Source: CAD feature listing. Evaluate the final solid. Frame: model axes, mm. Face numbers are marked on the shaded views. A direction names the side the tool comes from. Give positions to 0.01 mm unless a question says otherwise; leave off trailing zeros. Loops run counter-clockwise (first coordinate to the right, second up) from the corner with the lowest first, then second, coordinate; pieces in that order, holes last. Notation, with made-up numbers: M 59.5,42 L 94.5,42 A28 ccw 94.5,75 Z; hole C 82,59.25 d8. An arc over 180 degrees is marked long. Put each result on its own line as item: value.
from build123d import *

# Parameters (mm, degrees)
F1_DEPTH = 5
F3_DEPTH = 25


with BuildPart() as f1:
    # F0 (on Front) → F1 (new body)
    with BuildSketch(Plane.XZ):
        Polygon((48.04658, 78.242314), (-66.45342, 78.242314), (-66.45342, -34.757686), (-41.95342, -57.257686), (23.54658, -57.257686), (48.04658, -34.757686), align=None)
    extrude(amount=F1_DEPTH)

    # F2 (on face) → F3 (join)
    with BuildSketch(Plane.XZ.offset(5)):
        Polygon((23.54658, -57.257686), (48.04658, -34.757686), (48.04658, 78.242314), (-66.45342, 78.242314), (-66.45342, -34.757686), (-41.95342, -57.257686), align=None)
        Polygon((-61.45342, -32.560932), (-61.45342, 73.242314), (43.04658, 73.242314), (43.04658, -32.560932), (21.599003, -52.257686), (-40.005844, -52.257686), align=None, mode=Mode.SUBTRACT)
    extrude(amount=F3_DEPTH)


solid = f1.part
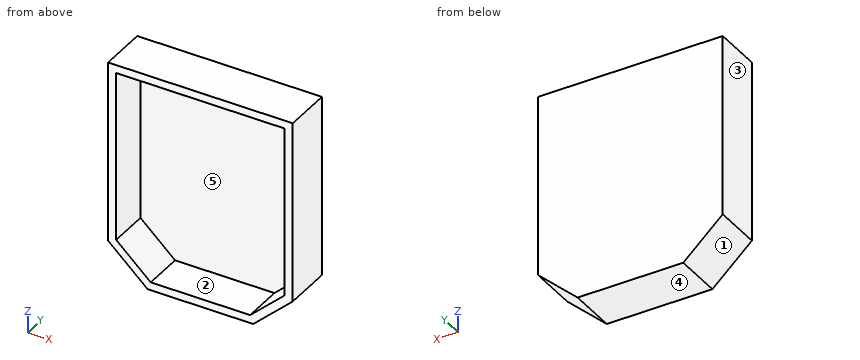
1. Section query A-A (y = -15.25). Output: boundary loops of the cut face in (x, z), plus the area to 3 significant figures.
Found:
outline: M -66.45,-34.76 L -41.95,-57.26 L 23.55,-57.26 L 48.05,-34.76 L 48.05,78.24 L -66.45,78.24 Z; hole M -61.45,-32.56 L -40.01,-52.26 L 21.6,-52.26 L 43.05,-32.56 L 43.05,73.24 L -61.45,73.24 Z
area: 2,270 mm^2
2. Section query B-B (x = -29). Output: boundary loops of the cut face in (y, z).
Found:
outline: M -30,-57.26 L 0,-57.26 L 0,78.24 L -30,78.24 L -30,73.24 L -5,73.24 L -5,-52.26 L -30,-52.26 Z
3. Contact query for a flat-ended pin moving along its axis: P1, Ø1, axis at x = 22.5, z = -10, coming from the -Y side. Output: stop coordinate, or through.
Found:
P1: y = -5
4. Material intervals for line 1 (Z direction, x = -39, y = -24.5); line 2 (X direction, y = -16, z = 23); line 3 (Y direction, x = -35, z = 60.5), sorted ascending. Write a range as from..to.
Found:
line 1: -57.26..-52.26, 73.24..78.24
line 2: -66.45..-61.45, 43.05..48.05
line 3: -5..0
5. Draft query along Z for the marked faces 3, 4 and 5. Return one class per face: pulls with the +Z half, pulls with the -Z half, needs draft (parallel to the pull), parting line crosses it, or undercut.
Found:
face 3: needs draft
face 4: pulls with the -Z half
face 5: undercut
6. Access query for the marked faces 1 and 2. Directions: +Z, -Z, +X, -X, +Y, -Y. A direction counts if a zero-diameter tool reaches every point of the face in a straight line with its end or side. Return the directions, or none.
Found:
face 1: -Z, -X, +Y, -Y
face 2: -Y
7. Section query C-C (z = 39). Output: boundary loops of the cut face in (x, y), plus the area to 4 significant figures.
Found:
outline: M -66.45,-30 L -61.45,-30 L -61.45,-5 L 43.05,-5 L 43.05,-30 L 48.05,-30 L 48.05,0 L -66.45,0 Z
area: 822.5 mm^2
